Can you work these out from the model? Positions are in its coordinate system, mm. Face numbers are marked on the shaded views. Coordinates: 2 decimals unless noted, no trailing zeros. Order: outer loops, then holes, each group sorted by start corner. A loop starts at its lowest first (then second) coordinate and runs counter-clockwise, first axis right, second up.
Autodesk Inventor part; units mm, degrees
ref_plane "YZ Plane" through (0, 0, 0) normal (1, 0, 0) x (0, 1, 0)
ref_plane "XZ Plane" through (0, 0, 0) normal (0, 1, 0) x (-1, 0, 0)
ref_plane "XY Plane" through (0, 0, 0) normal (0, 0, 1) x (1, 0, 0)
sketch "Sketch1" plane through (0, 0, 0) normal (0, 0, 1) x (1, 0, 0)
  line L0 (0, 0) -> (700, 0)
  line L1 (700, 0) -> (700, -400)
  line L2 (700, -400) -> (0, -400)
  line L3 (0, -400) -> (0, 0)
  dimension "d0" = 700
  dimension "d1" = 400
extrude "Extrusion1" add sketch "Sketch1" along normal blind 12
sketch "Sketch2" plane through (0, 0, 0) normal (0, 0, -1) x (-1, 0, 0)
  circle A0 centre (-350, -200) radius 80
  point P0 (0, 0)
  dimension "d4" = 160
extrude "Extrusion2" cut sketch "Sketch2" against normal blind 12
sketch "Sketch3" plane through (0, 0, 0) normal (0, 0, -1) x (-1, 0, 0)
  arc A0 (-430, -200) -> (-270, -200) centre (-350, -200) ccw
  line L0 (-270, -200) -> (-270, 0)
  line L1 (-430, -200) -> (-430, 0)
  line L2 (-265, 0) -> (-265, -200)
  arc A1 (-435, -200) -> (-265, -200) centre (-350, -200) ccw
  line L3 (-435, -200) -> (-435, 0)
  line L4 (-65, 0) -> (-65, -200)
  arc A2 (-635, -200) -> (-65, -200) centre (-350, -200) ccw
  line L5 (-635, -200) -> (-635, 0)
  line L6 (-60, 0) -> (-60, -200)
  arc A3 (-640, -200) -> (-60, -200) centre (-350, -200) ccw
  line L7 (-640, -200) -> (-640, 0)
  line L8 (-60, 0) -> (-65, 0)
  line L9 (-700, 0) -> (0, 0)
  line L10 (-430, 0) -> (-435, 0)
  line L11 (-635, 0) -> (-640, 0)
  line L12 (-265, 0) -> (-270, 0)
  dimension "d7" = 5
  dimension "d8" = 200
  dimension "d9" = 5
extrude "Extrusion3" add sketch "Sketch3" along normal blind 12 contours A0 L0 L9 L2 A1 L3 L1 | L5 A2 L4 L8 L6 A3 L7 L9
sketch "Sketch4" plane through (700, -400, 0) normal (1, 0, 0) x (0, 0, -1)
  line L0 (0, 0) -> (-12, 0)
  line L1 (0, 0) -> (-12, 0)
  line L2 (-12, 0) -> (-12, -90)
  line L3 (-12, -90) -> (0, -90)
  line L4 (0, -90) -> (0, 0)
  point P0 (0, 400)
  dimension "d12" = 90
extrude "Extrusion4" add sketch "Sketch4" against normal blind 700
sketch "Sketch5" plane through (700, 0, 12) normal (1, 0, 0) x (0, 0, -1)
  line L0 (12, 0) -> (0, 0)
  line L1 (0, 0) -> (88.8281, 0)
  line L2 (88.8281, 0) -> (88.8281, -90)
  line L3 (88.8281, -90) -> (0, -90)
  line L4 (0, -90) -> (0, 0)
  dimension "d15" = 90
extrude "Extrusion5" cut sketch "Sketch5" against normal blind 10000
sketch "Sketch6" plane through (0, -490, 0) normal (-1, 0, 0) x (0, 0, 1)
  line L0 (0, 290) -> (0, 400)
  line L1 (0, 400) -> (-31.175, 400)
  line L2 (-31.175, 400) -> (-31.175, 290)
  line L3 (-31.175, 290) -> (0, 290)
  line L4 (0, 290) -> (0, 400)
  point P0 (0, 490)
extrude "Extrusion6" cut sketch "Sketch6" against normal blind 500
sketch "Sketch7" plane through (0, 0, 0) normal (0, 0, -1) x (-1, 0, 0)
  circle A0 centre (-52.4557, -179.1018) radius 2.5
  circle A1 centre (-52.4557, -169.2668) radius 2.5
  point P0 (0, 0)
  dimension "d20" = 5
  dimension "d21" = 5
extrude "Extrusion7" add sketch "Sketch7" along normal blind 7
fillet "Fillet1" radius 2.5 2 edges at (54.9557, -169.2668, -7) (54.9557, -179.1018, -7)
fillet "Fillet2" radius 0.1 2 edges at (54.9557, -169.2668, 0) (54.9557, -179.1018, 0)
sketch "Sketch8" plane through (0, 0, 0) normal (0, 0, -1) x (-1, 0, 0)
  circle A0 centre (-63.0207, -108.7531) radius 10
  point P0 (0, 0)
  dimension "d26" = 20
extrude "Extrusion8" cut sketch "Sketch8" against normal blind 20
equation "\"BendRadius\" = Thickness"
equation "\"BendReliefWidth\" = Thickness"
equation "\"BendReliefDepth\" = 0.5 * Thickness"
equation "\"CornerReliefSize\" = 4 * Thickness"
equation "\"MinimumRemnant\" = 2 * Thickness"
equation "\"TransitionRadius\" = BendRadius"
equation "\"JacobiRadiusSize\" = BendRadius"
equation "\"GapSize\" = Thickness"
properties part number "base" material "Acetal Resin, White"
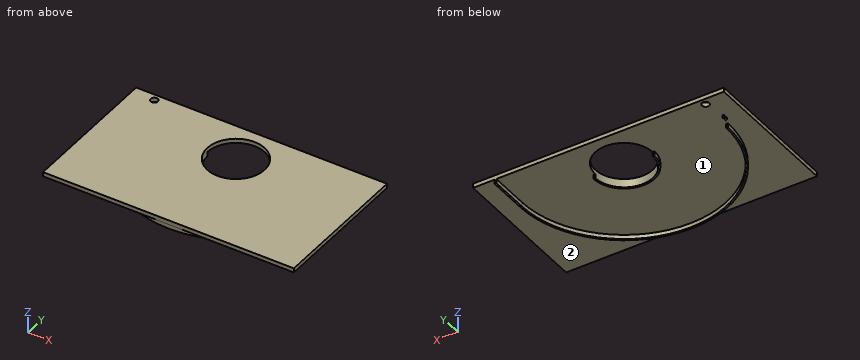
1. Imagine slicing it at D-D on y = -441.5. Please give me the cut outline in (x, z), then the cut area to 3 significant figures.
Completed:
outline: (0, 0) - (189.45, 0) - (189.45, -12) - (198.66, -12) - (198.66, 0) - (501.34, 0) - (501.34, -12) - (510.55, -12) - (510.55, 0) - (700, 0) - (700, 12) - (0, 12) - close
area: 8,620 mm2
2. I'm going to push flat-ended pins straight in: pin 1 (2.5 mm diameter, centred on x = 267, z = -6, fed in from +Y); pin 2 (1 mm diameter, centred on y = -438.5, z = -5.5, fed in from +X); pin 3 (3.5 mm diameter, centred on y = -134, z = -5.5, fed in from -X). Where does each tip first touch, or does it pass through?
Completed:
pin 1: stops at y = -200
pin 2: stops at x = 515.7
pin 3: stops at x = 635
3. Imagine slicing it at B-B on y = -211. Please give me the cut outline in (x, z), then the cut area to 3 significant figures.
Completed:
outline: (0, 0) - (60.21, 0) - (60.21, -12) - (65.21, -12) - (65.21, 0) - (265.71, 0) - (265.71, -12) - (270.76, -12) - (270.76, 12) - (0, 12) - close; (429.24, -12) - (434.29, -12) - (434.29, 0) - (634.79, 0) - (634.79, -12) - (639.79, -12) - (639.79, 0) - (700, 0) - (700, 12) - (429.24, 12) - close
area: 6,740 mm2
4. Imagine slicing it at A-A on x = 303. Please give me the cut outline in (y, z).
Completed:
outline: (-490, 0) - (-486.17, 0) - (-486.17, -12) - (-481.1, -12) - (-481.1, 0) - (-270.82, 0) - (-270.82, -12) - (-264.74, -12) - (-264.74, 12) - (-490, 12) - close; (-135.26, 0) - (-90, 0) - (-90, 12) - (-135.26, 12) - close
5. Please list where these lines run through material, in increasing order: probe 1 along Y at (x, z) = (350, -2.5); probe 2 along Y at (x, z) = (350, 3.25); probe 3 along X at (y, z) = (-205.5, -8.5).
Completed:
probe 1: y = -490 to -485, -285 to -280
probe 2: y = -490 to -280, -120 to -90
probe 3: x = 60.05 to 65.05, 265.18 to 270.19, 429.81 to 434.82, 634.95 to 639.95
6. Thinking about a two-plate mould opening in Y: for the marked faces 1 and 2, which applies, pulls with the +Y half, pulls with the -Y half, needs draft (parallel to the pull), parting line crosses it, or undercut?
Completed:
face 1: undercut
face 2: needs draft
7. Imagine slicing it at C-C on x = 162.5. Please give me the cut outline in (y, z), then the cut area to 3 significant figures.
Completed:
outline: (-490, 0) - (-421.23, 0) - (-421.23, -12) - (-414.64, -12) - (-414.64, 0) - (-90, 0) - (-90, 12) - (-490, 12) - close
area: 4,880 mm2
